Source: CAD feature listing. Evaluate the final solid. Frame: model axes, mm. A direction names the side the tool comes from. Give positions to 0.01 mm unless a question says otherwise; leave off trailing zeros. Write each loop counter-clockwise with the first axis right and the second up, starting at its lowest first coordinate (ties: lowest second). Pieces come first, ordered by that corner, then holes. Notation, with made-up numbers: (62, 62) - (75, 62) arc R34 cw to (75, 98) - close; hole circle Ø8 at (20.25, -33). An arc over 180 degrees is marked (long way). Answer as a JSON object with one key per item and string values. Group by question number.
from build123d import *

# Parameters (mm, degrees)
SKETCH1_W          = 882.65
SKETCH1_H          = 654.05
EXTRUDE1_DEPTH     = 4.7625
SKETCH2_R          = 6.35
CUT_EXTRUDE1_DEPTH = 5.7625
SKETCH3_W          = 177.8
SKETCH3_H          = 431.8
CUT_EXTRUDE2_DEPTH = 5.7625
FILLET1_R          = 25.4


with BuildPart() as part:
    # Sketch1 → Extrude1 (new body)
    with BuildSketch(Plane.XY):
        with Locations((-835.025, 91.6)):
            Rectangle(SKETCH1_W, SKETCH1_H)
    extrude(amount=EXTRUDE1_DEPTH)

    # Sketch2 → Cut-Extrude1 (cut, through all)
    with BuildSketch(Plane(origin=(0, 0, 0), x_dir=(-1, 0, 0), z_dir=(0, 0, -1))):
        with Locations((516.89, 254)):
            Circle(SKETCH2_R)
        with Locations((516.89, -70.8)):
            Circle(SKETCH2_R)
        with Locations((885.19, 254)):
            Circle(SKETCH2_R)
        with Locations((885.19, -70.8)):
            Circle(SKETCH2_R)
        with Locations((1253.49, -70.8)):
            Circle(SKETCH2_R)
        with Locations((1253.49, 254)):
            Circle(SKETCH2_R)
    extrude(amount=-CUT_EXTRUDE1_DEPTH, mode=Mode.SUBTRACT)

    # Sketch3 → Cut-Extrude2 (cut, through all)
    with BuildSketch(Plane.XY.offset(4.7625)):
        with Locations((-685.8, 91.6)):
            Rectangle(SKETCH3_W, SKETCH3_H)
    extrude(amount=-CUT_EXTRUDE2_DEPTH, mode=Mode.SUBTRACT)

    # Fillet1
    fillet1_edges = [part.edges().sort_by_distance(p)[0] for p in [
        (-596.9, 307.5, 2.38125),
        (-596.9, -124.3, 2.38125),
        (-774.7, -124.3, 2.38125),
        (-774.7, 307.5, 2.38125),
    ]]
    fillet(fillet1_edges, radius=FILLET1_R)


solid = part.part
Q1. Section B-B on y = 229. Return the cut outline in (x, z).
Q2. Section A-A on z = 3.2. Return the cut outline in (x, y) (3 decimals), then the cut area to 3 significant figures.
Q3. Draft query along X for faces 3 (the flat face through (-841, 96, 0)), 4 (the cylindrical face through (-604.54, -117.06, 2.35)), 5 (the cylindrical face through (-767.06, -117.06, 2.35)). Return one class per face: released by +X, released by -X, zero draft, split by the parting line, or undercut.
Q4. Reachability of faces 1 (the flat face through (-841, 96, 4.762)), 2 (the cylindrical face through (-604.14, 299.86, 2.35)) from +Z, -Z, +X, -X, +Y, -Y: full face, straight path, thin tool, end or side. Return the list, or none.
Q5. Ray query, probe 1 along Y at (x, z) = (-1253.49, 2.6) (3 decimals); probe 2 along X at (y, z) = (-63.5, 2.4); probe 3 along X at (y, z) = (249, 3.05). Return the intervals inside material, ascending. Write a range as [from, to].
Taken from the geometry:
{
 "1": {"outline": "(-1276.35, 0) - (-774.7, 0) - (-774.7, 4.76) - (-1276.35, 4.76) - close; (-596.9, 0) - (-393.7, 0) - (-393.7, 4.76) - (-596.9, 4.76) - close"},
 "2": {"outline": "(-1276.35, -235.425) - (-393.7, -235.425) - (-393.7, 418.625) - (-1276.35, 418.625) - close; hole circle Ø12.7 at (-1253.49, -70.8); hole circle Ø12.7 at (-1253.49, 254); hole circle Ø12.7 at (-885.19, -70.8); hole circle Ø12.7 at (-885.19, 254); hole (-774.7, -98.9) arc R25.4 ccw to (-749.3, -124.3) - (-622.3, -124.3) arc R25.4 ccw to (-596.9, -98.9) - (-596.9, 282.1) arc R25.4 ccw to (-622.3, 307.5) - (-749.3, 307.5) arc R25.4 ccw to (-774.7, 282.1) - close; hole circle Ø12.7 at (-516.89, -70.8); hole circle Ø12.7 at (-516.89, 254)", "area": "500,000 mm²"},
 "3": {"face 3": "zero draft", "face 4": "undercut", "face 5": "undercut"},
 "4": {"face 1": "+Z, +X, -X, +Y, -Y", "face 2": "+Z, -Z"},
 "5": {"probe 1": "y = [-235.425, -77.15], [-64.45, 247.65], [260.35, 418.625]", "probe 2": "x = [-1276.35, -774.7], [-596.9, -393.7]", "probe 3": "x = [-1276.35, -1257.4], [-1249.58, -889.1], [-881.28, -774.7], [-596.9, -520.8], [-512.98, -393.7]"}
}
